Design review of the part built by this model. Coordinates are the model's own, in mm. Face numbers are marked on the shaded views. Coordinates: 2 decimals unless noted, no trailing zeros. Write each loop counter-clockwise with the first axis right and the second up, starting at its lowest first coordinate (ties: lowest second). Pieces come first, ordered by that corner, then holes. Notation, with made-up numbers: M 2,-11 L 13,-11 A5 cw 13,-6 Z; hole C -21,88 d7. An arc over 180 degrees is marked long. Write item = value, one per line.
```python
from build123d import *

# Parameters (mm, degrees)
SKETCH1_R           = 4.5
BOSS_EXTRUDE1_DEPTH = 15
FILLET1_R           = 2
SCALE1_SCALE        = 1.5
SKETCH5_R           = 7.5
BOSS_EXTRUDE4_DEPTH = 10
FILLET6_R           = 330
SKETCH6_R           = 6.5
CUT_EXTRUDE1_DEPTH  = 12
BOSS_EXTRUDE5_DEPTH = 7
SKETCH8_R           = 1.75
BOSS_EXTRUDE6_DEPTH = 10
BOSS_EXTRUDE6_TAPER = 6
FILLET8_R           = 0.75
FILLET9_R           = 15


with BuildPart() as part:
    # Sketch1 → Boss-Extrude1 (new body)
    with BuildSketch(Plane(origin=(0, 0, 0), x_dir=(1, 0, 0), z_dir=(0, 1, 0))):
        with Locations(Location((0, 0, 0), (0, 0, 270))):
            Circle(SKETCH1_R)
    extrude(amount=BOSS_EXTRUDE1_DEPTH)

    # Fillet1
    fillet1_edges = [part.edges().sort_by_distance(p)[0] for p in [
        (0, 0, -4.5),
    ]]
    fillet(fillet1_edges, radius=FILLET1_R)


with BuildPart() as part_1:
    # Scale1: scaled about (0, 7.664895453, 0)
    add(part.part.scale(SCALE1_SCALE).moved(Location((0, -3.832447726, 0))))


with BuildPart() as body_2:
    # Sketch5 → Boss-Extrude4 (new body)
    with BuildSketch(Plane(origin=(0, 45, 0), x_dir=(1, 0, 0), z_dir=(0, 1, 0))):
        with Locations(Location((0, 0, 0), (0, 0, 270))):
            Circle(SKETCH5_R)
    extrude(amount=-BOSS_EXTRUDE4_DEPTH)


    add(part_1.part)  # loft1 joins it to this body
    # loft from a face of the part (loft1)
    loft([body_2.faces().sort_by_distance((0, 35, 0))[0], body_2.faces().sort_by_distance((0, 18.667552274, 0))[0]])

    # Fillet6
    # the kernel refuses this fillet: 330 mm, written as the material it takes off along each edge
    with BuildSketch(Plane(origin=(0, 35, 0), x_dir=(0, 0, 1), z_dir=(-1, 0, 0))) as fillet6_piece_1:
        with BuildLine():
            CenterArc((7.5 - FILLET6_R, FILLET6_R * 0.0229483370442), FILLET6_R, 357.370775756, 2.629224244)
            Line((7.5, FILLET6_R * 0.0229483370442), (7.5, 0))
            Line((7.5, 0), (7.5 - FILLET6_R * 0.00105269796789, -FILLET6_R * 0.0229241793765))
        make_face()
    revolve(axis=Axis((0, 35, 0), (0, 1, 0)), mode=Mode.SUBTRACT)

    # Fillet7: read off the stored shape, not the designer's step
    # Fillet7 outline → Fillet7 (revolve)
    with BuildSketch(Plane.XY):
        with BuildLine():
            ThreePointArc((6.75, 16.602201939), (6.773688822, 18.667008654), (6.844742817, 20.730728417))
            Line((6.844742817, 20.730728417), (6.75, 20.730728417))
            Line((6.75, 20.730728417), (6.75, 16.602201939))
        make_face()
    revolve(axis=Axis((0, 0, 0), (0, 1, 0)))

    # Sketch6 → Cut-Extrude1 (cut)
    with BuildSketch(Plane(origin=(0, 45, 0), x_dir=(1, 0, 0), z_dir=(0, 1, 0))):
        with Locations(Location((0, 0, 0), (0, 0, 270))):
            Circle(SKETCH6_R)
    extrude(amount=-CUT_EXTRUDE1_DEPTH, mode=Mode.SUBTRACT)

    # Sketch7 → Boss-Extrude5 (add)
    with BuildSketch(Plane(origin=(0, 33, 0), x_dir=(1, 0, 0), z_dir=(0, 1, 0))):
        with BuildLine():
            Line((-5.324488288, 3.728246836), (-4.505336244, 3.1546704))
            ThreePointArc((-4.505336244, 3.1546704), (-3.535331853, 4.213244437), (-2.32440044, 4.984692829))
            Line((-2.32440044, 4.984692829), (-2.747018701, 5.891000616))
            ThreePointArc((-2.747018701, 5.891000616), (-4.178119463, 4.97928888), (-5.324488288, 3.728246836))
        make_face()
    extrude(amount=BOSS_EXTRUDE5_DEPTH)

    # Sketch8 → Boss-Extrude6 (add)
    with BuildSketch(Plane.XZ.offset(3.832447727)):
        Circle(SKETCH8_R)
    extrude(amount=BOSS_EXTRUDE6_DEPTH, taper=BOSS_EXTRUDE6_TAPER)

    # Fillet8
    fillet8_edges = [body_2.edges().sort_by_distance(p)[0] for p in [
        (-0.698957647, -13.832447727, 0),
    ]]
    fillet(fillet8_edges, radius=FILLET8_R)

    # Fillet9
    # the kernel refuses this fillet: 15 mm, written as the material it adds along each edge
    with BuildSketch(Plane(origin=(0, -3.832447727, 0), x_dir=(1, 0, 0), z_dir=(0, 0, -1))) as fillet9_piece_1:
        with BuildLine():
            CenterArc((15.736552733, 10.428423347), FILLET9_R, 186, 42.247086963)
            Line((5.747758789, -0.761929442), (4.748879394, -1.880964721))
            ThreePointArc((4.748879394, -1.880964721), (3.75, -1.5), (1.75, -1.5))
            Line((1.75, -1.5), (0.258217157, -0.156792695))
            Line((0.258217157, -0.156792695), (0, 2.299979445))
            Line((0, 2.299979445), (0, 8.774445006))
            Line((0, 8.774445006), (0.818724302, 8.860496398))
        make_face()
    revolve(axis=Axis((0, -3.832447727, 0), (0, -1, 0)))


solid = body_2.part
```
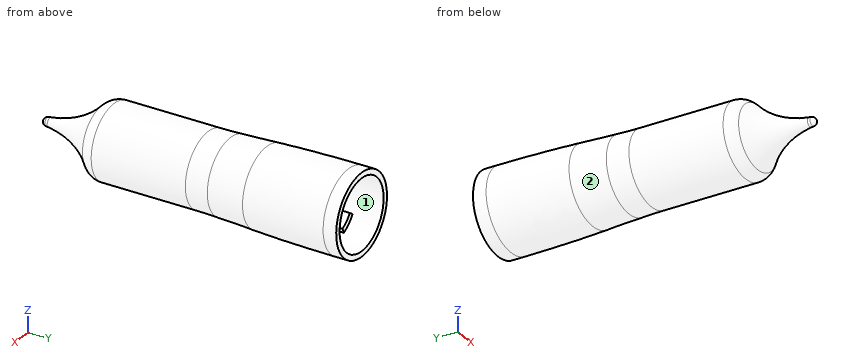
Q1. For P1, Ø1.4, axis at x = -4, z = -4, coming from the +Y side; P2, Ø6, axis at x = 5.5, y = 8.5, coming from the -Z side; P3, Ø3, axis at y = 6, z = -5.5, coming from the -X side, all flat-tipped, find the tip position at first contact; note any pin that passes through.
Check result:
P1 = 40
P2 = -6.27
P3 = -5.44
Q2. Consider section B-B, the plane y = -2.5. State the section outline as (x, z) points.
Check result:
outline = C 0,0 d12.49
Q3. Wall thickness on line 1 (X direction, y = 40.25, z = 0); line 2 (Z direction, x = 0, y = 41.75); line 3 (Z direction, x = -5.75, y = 37.5): over which ranges is each line inside the solid? List them lowest first.
Check result:
line_1 = -7.49 to -6.5, 6.5 to 7.49
line_2 = -7.5 to -6.5, 6.5 to 7.5
line_3 = -4.75 to -3.03, 3.03 to 4.75
Q4. Consider section A-A, the plane y = 23.5. State the section outline as (x, z) points.
Check result:
outline = C 0,0 d13.94
Q5. The part is to be moulded in two halves that separate along Z. For the marked faces 1 and 2, say which applies: +Z half, -Z half, draft (parallel to the pull), parting line (faces both ways), or undercut.
Check result:
face_1 = undercut
face_2 = parting line
